For this review, use the dimensioned drawing (mm, ordinates from the lowest corner) and the shaded views. A direction names the side the tool comes from. Give positions to 0.01 mm unless a question says otherwise; leave off trailing zeros. Write each loop counter-clockwise with the first axis right and the second up, starting at its lowest first coordinate (ties: lowest second). Pieces come first, ordered by that corner, then holes. Notation, with made-up numbers: (-27, 31) -> (-23, 31) arc R17 ccw to (-23, 55) -> close; hole circle Ø6 at (7, 26.5). An arc over 180 degrees is marked (long way). Write each question's results on one line, items separated by ' | '. Start each with the question number.
(1) For the marked faces 1 and 2, list the 3-axis set-ups (+Z, -Z, +X, -X, +Y, -Y) from which the entire face can be reached by the end or side of a thin tool; tool diameter is ignored.
(2) To check wall thickness, follow probe 1 along Z at (x, y) = (91, 22.5); probe 2 along Y at (x, z) = (94, 104.5) (1 decimal); probe 3 along X at (y, z) = (70, 46) (1 decimal). State the ranges of each line that lie inside material, in increasing order.
(3) Mouldability with a two-part tool opening along Y and no side actions: class the marked faces 3, 4 and 5 as released by +Y, released by -Y, zero draft, split by the parting line, or undercut.
(4) Clearance check with flat-ended pins moving along their axes: pin 1 (5 mm diameter, centred on y = 61, z = 35.5, fed in from -X); pin 2 (4 mm diameter, centred on x = 63.5, z = 105.5, fed in from -Y); pin 3 (4 mm diameter, centred on x = 95, y = 134.5, fed in from +Z). State where each tip first meets the part, or that it passes through.
(5) Take a section at D-D (z = 12). State the section outline as (x, y) points.
(6) Take a section at A-A (x = 74.5). State the section outline as (y, z) points (1 decimal), plus the area to 3 significant figures.
(7) Take a section at B-B (x = 94). State the section outline as (y, z) points (1 decimal).
(8) Take a section at C-C (y = 15). State the section outline as (x, z) points, plus the area to 3 significant figures.
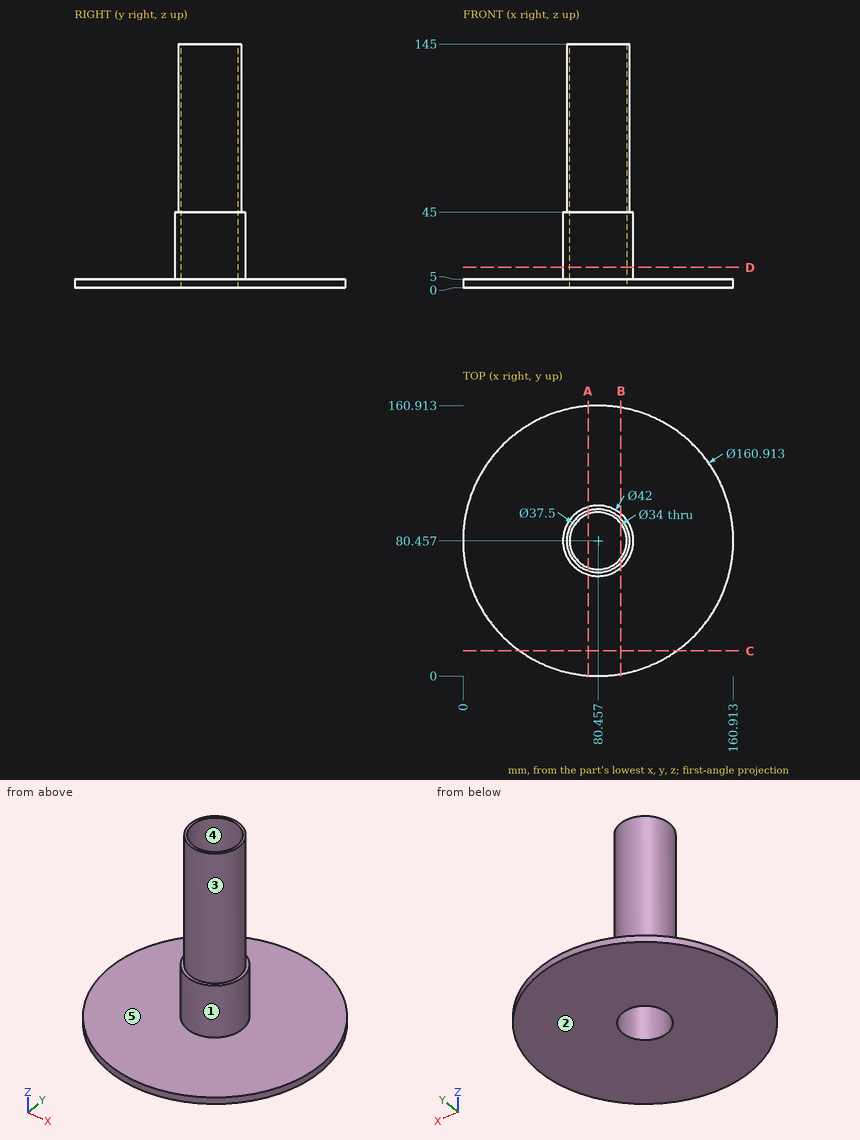
Report:
1) face 1: +Z | face 2: -Z, +X, -X, +Y, -Y
2) probe 1: 0 to 5 | probe 2: 67.5 to 70.2, 90.7 to 93.4 | probe 3: 64.9 to 67.1, 93.9 to 96
3) face 3: split by the parting line | face 4: undercut | face 5: zero draft
4) pin 1: x = 68.07 | pin 2: y = 69.15 | pin 3: z = 5
5) outline: circle Ø42 at (80.46, 80.46); hole circle Ø34 at (80.46, 80.46)
6) outline: (0.2, 0) -> (64.5, 0) -> (64.5, 145) -> (62.7, 145) -> (62.7, 45) -> (60.3, 45) -> (60.3, 5) -> (0.2, 5) -> close; (96.4, 0) -> (160.7, 0) -> (160.7, 5) -> (100.6, 5) -> (100.6, 45) -> (98.2, 45) -> (98.2, 145) -> (96.4, 145) -> close | area: 1,350 mm2
7) outline: (1.1, 0) -> (70.2, 0) -> (70.2, 145) -> (67.5, 145) -> (67.5, 45) -> (64.4, 45) -> (64.4, 5) -> (1.1, 5) -> close; (90.7, 0) -> (159.8, 0) -> (159.8, 5) -> (96.5, 5) -> (96.5, 45) -> (93.4, 45) -> (93.4, 145) -> (90.7, 145) -> close
8) outline: (33.67, 0) -> (127.24, 0) -> (127.24, 5) -> (33.67, 5) -> close | area: 468 mm2
